from build123d import *

# Parameters (mm, degrees)
F0_W     = 349.25
F0_H     = 127
F1_DEPTH = 19.05
F3_DEPTH = 12.7
F4_D     = 11.90625
F4_DEPTH = 34.925
F4_TIP   = 3.5769983726


# Not quite as in the source:
# - a pattern or mirror of a feature is missing from the dataset's text; its kind, count and spacing are read off the source's solid


with BuildPart() as f1:
    # F0 (on Front) → F1 (new body)
    with BuildSketch(Plane.XZ):
        Rectangle(F0_W, F0_H)
    extrude(amount=F1_DEPTH)

    # F2 (on face) → F3 (cut)
    with BuildSketch(Plane(origin=(-174.625, 0, 0), x_dir=(0, -1, 0), z_dir=(-1, 0, 0))):
        Polygon((19.05, -47.625), (19.05, -28.575), (6.35, -25.4085343639), (6.35, -50.7914656361), align=None)
        Polygon((19.05, -9.525), (19.05, 9.525), (6.35, 12.6914656361), (6.35, -12.6914656361), align=None)
        Polygon((19.05, 28.575), (19.05, 47.625), (6.35, 50.7914656361), (6.35, 25.4085343639), align=None)
    f3 = extrude(amount=-F3_DEPTH, mode=Mode.SUBTRACT)

    # F3_copies: F3 across plane
    add(f3.mirror(Plane(origin=(0, 0, 0), x_dir=(0, 0, 1), z_dir=(1, 0, 0))), mode=Mode.SUBTRACT)

    # F4
    with Locations(Plane(origin=(0, 0, 0), x_dir=(1, 0, 0), z_dir=(0, 1, 0))):
        with Locations((0, 0)):
            Hole(F4_D / 2, depth=F4_DEPTH)
            with Locations((0, 0, -(F4_DEPTH + F4_TIP / 2))):  # 118° drill point
                Cone(0, F4_D / 2, F4_TIP, mode=Mode.SUBTRACT)


solid = f1.part
For this review, take the finished solid that the model builds, in its own axes (mm). A direction names the side the tool comes from. Round coordinates to 2 decimals unless told otherwise and drop trailing zeros. Write each loop counter-clockwise with the first axis right and the second up, starting at its lowest first coordinate (ties: lowest second). Pieces come first, ordered by that corner, then holes. Notation, with made-up numbers: (-11, 24.25) - (46, 24.25) arc R19 cw to (46, 38.25) - close; hole circle Ø2 at (-9, 35). An arc over 180 degrees is marked (long way). Write item = value, one per line. Start each with the question number.
1. Consider section B-B on z = 0. State the section outline as (x, y) points (3 decimals), plus the area to 3 significant figures.
2. Consider section A-A on x = 0. State the section outline as (y, z) points.
3. For pin 1 Ø6.5 at (x, z) = (-168.5, 3.5) entering from -Y; pin 2 Ø6.5 at (y, z) = (-10.5, -37) entering from +X (3 decimals); pin 3 Ø4 at (y, z) = (-12, -2) entering from -X (3 decimals), all flat-tipped, find the tip position at first contact; note any pin that passes through.
4. Consider section C-C on z = -44.5. State the section outline as (x, y) points (3 decimals), plus the area to 3 significant figures.
5. For faces 1 (the face through (4.724, -9.658, 3.622)), 2 (the face through (-161.925, -13, 38)), 3 (the face through (168, -6.35, 38)), list the 3-axis set-ups (+Z, -Z, +X, -X, +Y, -Y) from which the entire face can be reached by the end or side of a thin tool; tool diameter is ignored.
6. Draft analysis for pull direction Y (two halves, no side actions). For faces 4 (the face through (174.625, -5, -1)), 5 (the face through (168.364, -12.789, 49.186)), 6 (the face through (-2, -19.05, 15)), state which applies: released by +Y, released by -Y, zero draft, split by the parting line, or undercut.
7. Wall thickness on L1, parallel to Z at x = 0, y = -7.25; L2, parallel to Z at x = -1, y = -16.75: over which ranges is each line inside the solid? List them lowest first.
Evaluation:
q1.outline = (-174.625, -6.35) - (-161.925, -6.35) - (-161.925, -19.05) - (-5.953, -19.05) - (-5.953, 0) - (-174.625, 0) - close; (5.953, -19.05) - (161.925, -19.05) - (161.925, -6.35) - (174.625, -6.35) - (174.625, 0) - (5.953, 0) - close
q1.area = 6,100 mm2
q2.outline = (-19.05, -63.5) - (0, -63.5) - (0, -5.95) - (-19.05, -5.95) - close; (-19.05, 5.95) - (0, 5.95) - (0, 63.5) - (-19.05, 63.5) - close
q3.pin_1 = -6.35
q3.pin_2 = 161.925
q3.pin_3 = -161.925
q4.outline = (-174.625, -6.35) - (-161.925, -6.35) - (-161.925, -19.05) - (161.925, -19.05) - (161.925, -6.35) - (174.625, -6.35) - (174.625, 0) - (-174.625, 0) - close
q4.area = 6,330 mm2
q5.face_1 = +Y, -Y
q5.face_2 = -X
q5.face_3 = +X
q6.face_4 = zero draft
q6.face_5 = undercut
q6.face_6 = released by -Y
q7.L1 = -63.5 to -5.95, 5.95 to 63.5
q7.L2 = -63.5 to -5.87, 5.87 to 63.5
